Input: part model. Units: mm. Frame: model coordinates. A direction names the side the tool comes from. Give positions to 0.01 mm unless a question says otherwise; leave off trailing zeros. Order: outer loops, then holes, each group sorted by start corner. A loop starts at its lowest first (then second) coordinate and runs counter-clockwise, first axis right, second up. Notation, with made-up numbers: (63, -4.5) -> (84, -4.5) arc R11 ccw to (84, 2.5) -> close; hole circle Ø4 at (13.5, 40). An arc over 180 degrees is marked (long way). Use a Markdown table: item, result. Add a question column.
from build123d import *

# Parameters (mm, degrees)
SKETCH1_R           = 2.2
BOSS_EXTRUDE1_DEPTH = 3
SKETCH3_W           = 19.05
SKETCH3_H           = 19.05
SKETCH3_R           = 2.2
SKETCH3_R_2         = 5
CUT_EXTRUDE1_DEPTH  = 83.785868359
CUT_EXTRUDE2_DEPTH  = 10


with BuildPart() as part:
    # Sketch1 → Boss-Extrude1 (new body)
    with BuildSketch(Plane(origin=(0, 0, 0), x_dir=(1, 0, 0), z_dir=(0, 1, 0))):
        Polygon((-58.5, 19.5), (-58.5, 58.5), (-19.5, 58.5), (-19.5, 55.5), (19.5, 55.5), (19.5, 58.5), (58.5, 58.5), (58.5, 19.5), (55.5, 19.5), (55.5, -19.5), (58.5, -19.5), (58.5, -58.5), (19.5, -58.5), (19.5, -55.5), (-19.5, -55.5), (-19.5, -58.5), (-58.5, -58.5), (-58.5, -19.5), (-55.5, -19.5), (-55.5, 19.5), align=None)
        with Locations(Location((-37.5, 37.5, 0), (0, 0, 270))):
            Circle(SKETCH1_R, mode=Mode.SUBTRACT)
        with Locations(Location((37.5, 37.5, 0), (0, 0, 270))):
            Circle(SKETCH1_R, mode=Mode.SUBTRACT)
        with Locations(Location((37.5, -37.5, 0), (0, 0, 270))):
            Circle(SKETCH1_R, mode=Mode.SUBTRACT)
        with Locations(Location((-37.5, -37.5, 0), (0, 0, 270))):
            Circle(SKETCH1_R, mode=Mode.SUBTRACT)
    extrude(amount=BOSS_EXTRUDE1_DEPTH)

    # Sketch3 → Cut-Extrude1 (cut, through all)
    with BuildSketch(Plane(origin=(0, 3, 0), x_dir=(1, 0, 0), z_dir=(0, 1, 0))):
        with Locations((20.32, 30.48)):
            Rectangle(SKETCH3_W, SKETCH3_H)
        with Locations((20.32, 10.16)):
            Rectangle(SKETCH3_W, SKETCH3_H)
        with Locations((20.32, -10.16)):
            Rectangle(SKETCH3_W, SKETCH3_H)
        with Locations((20.32, -30.48)):
            Rectangle(SKETCH3_W, SKETCH3_H)
        with Locations((0, -30.48)):
            Rectangle(SKETCH3_W, SKETCH3_H)
        with Locations((0, -10.16)):
            Rectangle(SKETCH3_W, SKETCH3_H)
        with Locations((0, 10.16)):
            Rectangle(SKETCH3_W, SKETCH3_H)
        with Locations((0, 30.48)):
            Rectangle(SKETCH3_W, SKETCH3_H)
        with Locations((-20.32, 30.48)):
            Rectangle(SKETCH3_W, SKETCH3_H)
        with Locations((-20.32, 10.16)):
            Rectangle(SKETCH3_W, SKETCH3_H)
        with Locations((-20.32, -10.16)):
            Rectangle(SKETCH3_W, SKETCH3_H)
        with Locations((-20.32, -30.48)):
            Rectangle(SKETCH3_W, SKETCH3_H)
        with Locations((-37.5, 37.5)):
            Circle(SKETCH3_R)
        with Locations((-41.29, 28.56)):
            Rectangle(SKETCH3_W, SKETCH3_H)
        with Locations((-41.29, 8.24)):
            Rectangle(SKETCH3_W, SKETCH3_H)
        with Locations((37.5, 37.5)):
            Circle(SKETCH3_R)
        with Locations((41.29, 28.56)):
            Rectangle(SKETCH3_W, SKETCH3_H)
        with Locations((41.29, 8.24)):
            Rectangle(SKETCH3_W, SKETCH3_H)
        with Locations(Location((-43.718159869, -11.432070866, 0), (0, 0, 270))):
            Circle(SKETCH3_R_2)
        with Locations(Location((-43.718159869, -26.672070866, 0), (0, 0, 270))):
            Circle(SKETCH3_R_2)
        with Locations(Location((43.901840131, -11.432070866, 0), (0, 0, 270))):
            Circle(SKETCH3_R_2)
        with Locations(Location((43.901840131, -26.672070866, 0), (0, 0, 270))):
            Circle(SKETCH3_R_2)
    extrude(amount=-CUT_EXTRUDE1_DEPTH, mode=Mode.SUBTRACT)

    # Sketch4 → Cut-Extrude2 (cut)
    with BuildSketch(Plane(origin=(0, 3, 0), x_dir=(1, 0, 0), z_dir=(0, 1, 0))):
        Polygon((-31.765, -1.285), (-29.845, -1.285), (-29.845, -40.005), (29.845, -40.005), (29.845, -1.285), (50.815, -1.285), (50.815, 38.085), (29.845, 38.085), (10.795, 40.005), (-10.795, 40.005), (-29.845, 38.085), (-31.765, 38.085), (-50.815, 19.035), (-50.815, 17.765), align=None)
    extrude(amount=-CUT_EXTRUDE2_DEPTH, mode=Mode.SUBTRACT)


solid = part.part
Q1. Ray query, line 1 (X direction, y = 2.35, z = 37.5) (3 decimals); line 2 (Z direction, x = -50, y = 0.2) (3 decimals); line 3 (X direction, y = 1.4, z = -4.5) (3 decimals). Return the intervals inside material, ascending.
Q2. Draft query along Z for faces 1 (the flat face through (58.5, 1, -39)), 2 (the flat face through (39, 1, -58.5)), 3 (the flat face through (33, 2, -38.085)). Return one class per face: +Z half, -Z half, draft (parallel to the pull), parting line (faces both ways), or undercut.
Q3. Section query B-B (x = 37.5). Return loops of the section in (y, z) (3 decimals), plus the area to 3 significant figures.
Q4. Access query for faces 4 (the flat face through (-40, 2, 1.285)), 5 (the flat face through (-19.5, 1, -57)), 6 (the flat face through (0, 1, 55.5)), 7 (the flat face through (57, 1, -19.5)). Directions: +Z, -Z, +X, -X, +Y, -Y. A direction counts if a zero-diameter tool reaches every point of the face in a straight line with its end or side. Return the directions, or none.
Q5. Section query D-D (z = 24.5). Return loops of the section in (x, y) (3 decimals).
Q6. First-contact query: pin 1 (1.5 mm diameter, centred on x = -4, y = 1, fed in from +Z); pin 2 (2.5 mm diameter, centred on x = -37.5, z = 37.5, fed in from +Y). Flat tips, straight axial feed; report the tip coordinate or a pass-through.
Q7. Section query C-C (z = 37.5). Return loops of the section in (x, y) (3 decimals).
Q8. Section query A-A (z = -26.5). Return loops of the section in (x, y) (3 decimals).
Solution:
| question | item | result |
|---|---|---|
| 1 | line 1 | x = -58.5 to -39.7, -35.3 to -29.845, 29.845 to 35.3, 39.7 to 58.5 |
| 1 | line 2 | z = -58.5 to -38.085, 1.285 to 58.5 |
| 1 | line 3 | x = -55.5 to -50.815, 50.815 to 55.5 |
| 2 | face 1 | draft |
| 2 | face 2 | -Z half |
| 2 | face 3 | undercut |
| 3 | outline | (0, -58.5) -> (3, -58.5) -> (3, -39.7) -> (0, -39.7) -> close; (0, 1.285) -> (3, 1.285) -> (3, 35.3) -> (0, 35.3) -> close; (0, 39.7) -> (3, 39.7) -> (3, 58.5) -> (0, 58.5) -> close |
| 3 | area | 215 mm² |
| 4 | face 4 | +Y, -Y |
| 4 | face 5 | -Z, +Y, -Y |
| 4 | face 6 | +Z, +Y, -Y |
| 4 | face 7 | +X, +Y, -Y |
| 5 | outline | (-58.5, 0) -> (-48.222, 0) -> (-48.222, 3) -> (-58.5, 3) -> close; (-39.215, 0) -> (-29.845, 0) -> (-29.845, 3) -> (-39.215, 3) -> close; (29.845, 0) -> (39.398, 0) -> (39.398, 3) -> (29.845, 3) -> close; (48.405, 0) -> (58.5, 0) -> (58.5, 3) -> (48.405, 3) -> close |
| 6 | pin 1 | stops at z = 55.5 |
| 6 | pin 2 | passes through |
| 7 | outline | (-58.5, 0) -> (-39.7, 0) -> (-39.7, 3) -> (-58.5, 3) -> close; (-35.3, 0) -> (-29.845, 0) -> (-29.845, 3) -> (-35.3, 3) -> close; (29.845, 0) -> (35.3, 0) -> (35.3, 3) -> (29.845, 3) -> close; (39.7, 0) -> (58.5, 0) -> (58.5, 3) -> (39.7, 3) -> close |
| 8 | outline | (-58.5, 0) -> (-50.815, 0) -> (-50.815, 3) -> (-58.5, 3) -> close; (50.815, 0) -> (58.5, 0) -> (58.5, 3) -> (50.815, 3) -> close |
